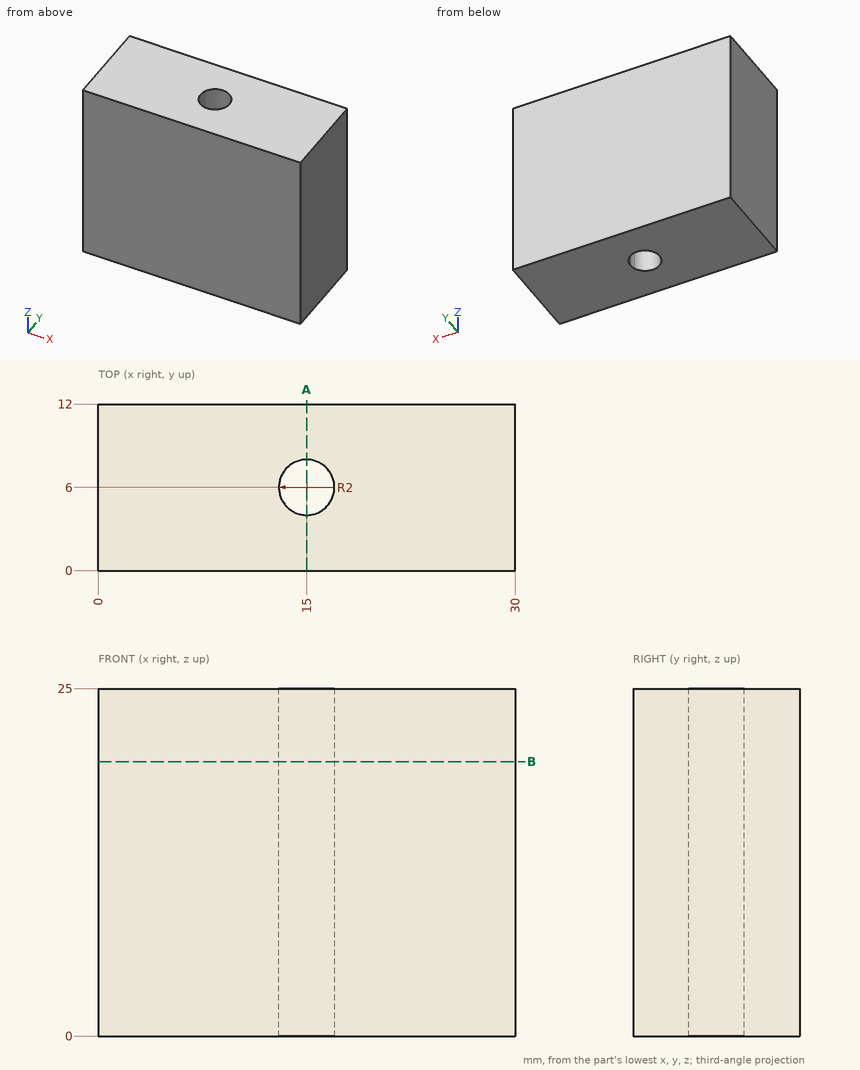
Input: dimensioned drawing with shaded views. Units: mm. Origin: part minimum x, y, z. Round coordinates to 2 decimals unless told otherwise and drop trailing zeros. Loops run counter-clockwise (first coordinate to the right, second up) from the corner with the lowest first, then second, coordinate; pieces in that order, holes last.
1) Section query A-A on x = 15. Return the cut outline in (y, z), plus the area to 3 significant figures.
Ans:
outline: (0, 0) - (4, 0) - (4, 25) - (0, 25) - close; (8, 0) - (12, 0) - (12, 25) - (8, 25) - close
area: 200 mm2
2) Material intervals for line 1 (Y direction, x = 15, z = 10.5); line 2 (X direction, y = 6.75, z = 12.75); line 3 (X direction, y = 4.5, z = 22.75), sorted ascending.
Ans:
line 1: y = 0 to 4, 8 to 12
line 2: x = 0 to 13.15, 16.85 to 30
line 3: x = 0 to 13.68, 16.32 to 30
3) Section query B-B on z = 19.75. Return the cut outline in (x, y), plus the area to 3 significant figures.
Ans:
outline: (0, 0) - (30, 0) - (30, 12) - (0, 12) - close; hole circle Ø4 at (15, 6)
area: 347 mm2
